Geometry check sheet. Reference: the model listing, model coordinates, mm. Round coordinates to 2 decimals unless told otherwise and drop trailing zeros. Order: outer loops, then holes, each group sorted by start corner. A loop starts at its lowest first (then second) coordinate and runs counter-clockwise, first axis right, second up.
(1) Cross-section at A-A on z = 0.7. Count the separate pieces of the cut face and the enclosed holes in it, and give its area (3 significant figures).
(2) Thickness scan on L1, parallel to X at y = -289.5, z = 3; L2, parallel to X at y = -319.5, z = 1.2; L3, parallel to Y at x = -232, z = 2.85. Record the ranges inside material, lowest first.
(3) Gauge pin test, flat end, axial feed: P1, Ø1.2, axis at y = -14.5, z = 1.5, coming from the +X side. Record the tip position at first contact, or that the pin passes through.
(4) Cross-section at B-B on y = -39. Enter the section's corners in (x, z), and give its area (3 significant figures).
from build123d import *

# Parameters (mm, degrees)
EXTRUDE_1_DEPTH     = 4
SKETCH_2_W          = 11.5
SKETCH_2_H          = 6.8
CUT_EXTRUDE_1_DEPTH = 747.201380326
SKETCH_3_R          = 3.25
CUT_EXTRUDE_2_DEPTH = 747.201380326
SKETCH_4_R          = 3.1
CUT_EXTRUDE_3_DEPTH = 747.201380326


with BuildPart() as part:
    # Эскиз1 → Бобышка-Вытянуть1 (new body)
    with BuildSketch(Plane.XY):
        Polygon((-669.5, 2.95), (-26.041378029, 2.95), (59.5, 88.491378029), (59.5, 329.5), (-669.5, 329.5), align=None)
    extrude(amount=EXTRUDE_1_DEPTH)

    # Эскиз2 → Вырез-Вытянуть1 (cut, through all)
    with BuildSketch(Plane(origin=(0, 0, 0), x_dir=(-1, 0, 0), z_dir=(0, 0, -1))):
        with Locations((65.75, 15.42)):
            Rectangle(SKETCH_2_W, SKETCH_2_H)
        with Locations((82.75, 15.42)):
            Rectangle(SKETCH_2_W, SKETCH_2_H)
        with Locations((527.25, 15.42)):
            Rectangle(SKETCH_2_W, SKETCH_2_H)
        with Locations((544.25, 15.42)):
            Rectangle(SKETCH_2_W, SKETCH_2_H)
    extrude(amount=-CUT_EXTRUDE_1_DEPTH, mode=Mode.SUBTRACT)

    # Эскиз3 → Вырез-Вытянуть2 (cut, through all)
    with BuildSketch(Plane(origin=(0, 0, 0), x_dir=(-1, 0, 0), z_dir=(0, 0, -1))):
        with Locations((232, 289.5)):
            Circle(SKETCH_3_R)
        with Locations((378, 289.5)):
            Circle(SKETCH_3_R)
    extrude(amount=-CUT_EXTRUDE_2_DEPTH, mode=Mode.SUBTRACT)

    # Эскиз4 → Вырез-Вытянуть3 (cut, through all)
    with BuildSketch(Plane(origin=(0, 0, 0), x_dir=(-1, 0, 0), z_dir=(0, 0, -1))):
        with Locations((-49.5, 319.5)):
            Circle(SKETCH_4_R)
        with Locations((659.5, 319.5)):
            Circle(SKETCH_4_R)
    extrude(amount=-CUT_EXTRUDE_3_DEPTH, mode=Mode.SUBTRACT)


with BuildPart() as body_2:
    # Зеркальное отражение1: mirrored copy
    add(part.part.mirror(Plane.ZX))


solid = body_2.part
Found:
1. separate pieces: 1
1. enclosed holes: 8
1. area: 234,000 mm2
2. L1: x = -669.5 to -381.25, -374.75 to -235.25, -228.75 to 59.5
2. L2: x = -669.5 to -662.6, -656.4 to 46.4, 52.6 to 59.5
2. L3: y = -329.5 to -292.75, -286.25 to -2.95
3. P1: stops at x = -13.89
4. outline: (-669.5, 0) - (10.01, 0) - (10.01, 4) - (-669.5, 4) - close
4. area: 2,720 mm2
